CAD build for the part. Positions are in the model's coordinates, mm. Face numbers are marked on the shaded views. A direction names the side the tool comes from. Coordinates: 2 decimals unless noted, no trailing zeros. Order: outer loops, then holes, each group sorted by start corner. A loop starts at its lowest first (then second) coordinate and runs counter-clockwise, first axis right, second up. Notation, with made-up numbers: (48.5, 15) - (85.5, 15) arc R16 cw to (85.5, 39) - close; hole circle Ø8 at (80.25, 39.5). An arc over 180 degrees is marked (long way). Write each question's results on one line, items separated by ' | '. Start each with the question number.
Q1. Band-saw the part on D-D, the plane x = 8. Write the cut outline in (y, z), then the cut area to 3 significant figures.
Q2. Pull direction Z, two halves, no side cores. Call the marked faces 4, 5, 6 and 7: released by +Z, released by -Z, zero draft, split by the parting line, or undercut.
Q3. Band-saw the part on B-B, the plane y = 7.5. Write the cut outline in (x, z), then the cut area to 3 significant figures.
Q4. Band-saw the part on C-C, the plane z = 27.5. Write the cut outline in (x, y), then the cut area to 3 significant figures.
Q5. Which spindle directions (+Z, -Z, +X, -X, +Y, -Y) get a long thin tool onto all of the face, cutting with end or side? Do the marked faces 1, 2 and 3. Say none if no direction does.
Q6. Pin check, flat tips, straight feed: P1, Ø15, axis at y = 60, z = 19.5, coming from the +X side; P2, Ø25, axis at x = 37.5, z = 36.5, coming from the +Y side. Stop position of each tip, or through.
Q7. Wall check: probe 1 along Y at (x, z) = (13.5, 25.5); probe 2 along Z at (x, y) = (62.5, 12.5); probe 3 along Y at (x, z) = (31.5, 41.5). Give the ranges that are in metal, low to high.
Q8. Band-saw the part on A-A, the plane z = 18. Write the cut outline in (x, y), then the cut area to 3 significant figures.
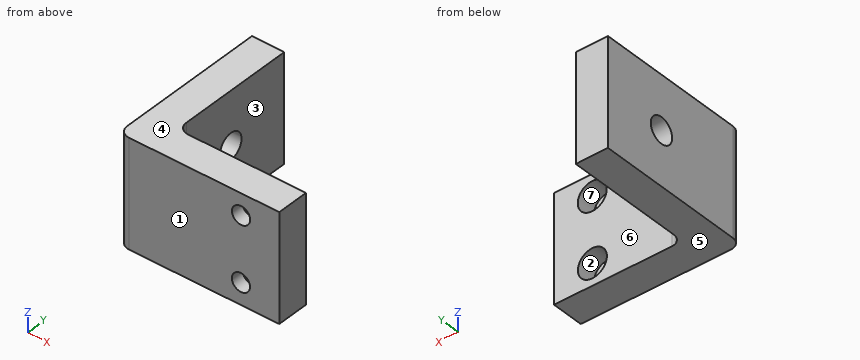
```python
from build123d import *

# Parameters (mm, degrees)
F0_W           = 15.0410700589
F0_H           = 23.9910148084
F1_DEPTH       = 50
F3_D           = 12
F5_D           = 8.5
F5_DEPTH       = 15
F5_CBORE_D     = 13.5
F5_CBORE_DEPTH = 9
F5_TIP         = 2.5536576309


with BuildPart() as f1:
    # F0 (on Top) → F1 (new body)
    with BuildSketch(Plane.XY):
        with BuildLine():
            Line((0, 39.0400364995), (0, 5))
            ThreePointArc((0, 5), (1.4644660941, 1.4644660941), (5, 0))
            Line((5, 0), (52.6695400476, 0))
            Line((52.6695400476, 0), (52.6695400476, 6.0573876835))
            Line((52.6695400476, 6.0573876835), (50.1525513828, 6.0573876835))
            Line((50.1525513828, 6.0573876835), (50.1525513828, 15.0117706507))
            Line((50.1525513828, 15.0117706507), (20.0410700589, 15.0117706507))
            ThreePointArc((20.0410700589, 15.0117706507), (16.505536153, 16.4762367448), (15.0410700589, 20.0117706507))
            Line((15.0410700589, 20.0117706507), (15.0410700589, 25.0367524475))
            Line((15.0410700589, 25.0367524475), (15.0410700589, 39.0400364995))
            Line((15.0410700589, 39.0400364995), (0, 39.0400364995))
        make_face()
        Polygon((0, 45.056425035), (0, 39.0400364995), (15.0410700589, 39.0400364995), (15.0410700589, 45.056425035), (15.0410700589, 51.040943712), (0, 51.040943712), align=None)
        Polygon((52.6695400476, 6.0573876835), (52.6695400476, 0), (56.8805225194, 0), (61.0882826149, 0), (61.0882826149, 6.0573876835), (63.6130347848, 6.0573876835), (63.6130347848, 15.0117706507), (50.1525513828, 15.0117706507), (50.1525513828, 6.0573876835), align=None)
        with Locations((7.5205350295, 63.0364511162)):
            Rectangle(F0_W, F0_H)
        Polygon((0, 75.1270577312), (0, 75.0319585204), (15.0410700589, 75.0319585204), align=None)
        Polygon((61.0882826149, 6.0573876835), (61.0882826149, 0), (74.9153345823, 0), (74.9153345823, 15.0117706507), (63.6130347848, 15.0117706507), (63.6130347848, 6.0573876835), align=None)
    extrude(amount=F1_DEPTH)

    # F3 (through all)
    with Locations(Plane(origin=(0, 0, 0), x_dir=(0, 1, 0), z_dir=(-1, 0, 0))):
        with Locations((45.0686700642, -25.0693447888)):
            Hole(F3_D / 2)

    # F5
    with Locations(Plane(origin=(0, 15.0117706507, 0), x_dir=(-1, 0, 0), z_dir=(0, 1, 0))):
        with Locations((-57.1296028793, 40.0831848383), (-57.0615939796, 10.0682657212)):
            CounterBoreHole(F5_D / 2, F5_CBORE_D / 2, F5_CBORE_DEPTH, depth=F5_DEPTH)
            with Locations((0, 0, -(F5_DEPTH + F5_TIP / 2))):  # 118° drill point
                Cone(0, F5_D / 2, F5_TIP, mode=Mode.SUBTRACT)


solid = f1.part
```
Results below:
1) outline: (0, 0) - (75.08, 0) - (75.08, 50) - (0, 50) - close; hole circle Ø12 at (45.07, 25.07) | area: 3,640 mm²
2) face 4: released by +Z | face 5: released by -Z | face 6: zero draft | face 7: undercut
3) outline: (0, 0) - (74.92, 0) - (74.92, 50) - (0, 50) - close; hole circle Ø13.5 at (57.06, 10.07); hole circle Ø13.5 at (57.13, 40.08) | area: 3,460 mm²
4) outline: (0, 5) arc R5 ccw to (5, 0) - (74.92, 0) - (74.92, 15.01) - (20.04, 15.01) arc R5 cw to (15.04, 20.01) - (15.04, 39.58) - (0, 39.58) - close; (0, 50.55) - (15.04, 50.55) - (15.04, 75.03) - (0, 75.13) - close | area: 1,860 mm²
5) face 1: +Z, -Z, +X, -X, -Y | face 2: +Y | face 3: +Z, -Z, +X, +Y
6) P1: stops at x = 15.04 | P2: stops at y = 15.01
7) probe 1: y = 0 to 39.08, 51.05 to 75.04 | probe 2: z = 0 to 6.07, 14.07 to 35.99, 44.17 to 50 | probe 3: y = 0 to 15.01
8) outline: (0, 5) arc R5 ccw to (5, 0) - (74.92, 0) - (74.92, 15.01) - (20.04, 15.01) arc R5 cw to (15.04, 20.01) - (15.04, 75.03) - (0, 75.13) - close | area: 2,030 mm²
